```python
from build123d import *

# Parameters (mm, degrees)
F0_W     = 50.8
F0_H     = 50.8
F1_DEPTH = 6.35
F2_W     = 6.3624648929
F2_H     = 50.8
F2_W_2   = 6.35
F3_DEPTH = 44.45
F4_R     = 5.08
F5_DEPTH = 6.35
F7_DEPTH = 148.336
F8_R     = 7.9375
F9_DEPTH = 94.742


with BuildPart() as f1:
    # F0 (on Front) → F1 (new body)
    with BuildSketch(Plane.XZ):
        with Locations((-25.4, 25.4)):
            Rectangle(F0_W, F0_H)
    extrude(amount=F1_DEPTH)

    # F2 (on face) → F3 (join)
    with BuildSketch(Plane.XZ.offset(6.35)):
        with Locations((-47.6187675536, 25.4)):
            Rectangle(F2_W, F2_H)
        with Locations((-3.175, 25.4)):
            Rectangle(F2_W_2, F2_H)
    extrude(amount=F3_DEPTH)

    # F4
    f4_edges = [f1.edges().sort_by_distance(p)[0] for p in [
        (-6.35, -6.35, 25.4),
        (-50.8, 0, 25.4),
        (-44.437535, -6.35, 25.4),
        (0, 0, 25.4),
    ]]
    fillet(f4_edges, radius=F4_R)

    # F5 (add): faces of the model
    f5_faces = [f1.faces().sort_by_distance(p)[0] for p in [
        (-47.6187675536, -50.8, 25.4),
        (-3.175, -50.8, 25.4),
        (-47.6187675536, -50.8, 25.4),
        (-3.175, -50.8, 25.4),
    ]]
    extrude(f5_faces, amount=F5_DEPTH)

    # F6 (on face) → F7 (cut)
    with BuildSketch(Plane(origin=(-50.8, 0, 0), x_dir=(0, -1, 0), z_dir=(-1, 0, 0))):
        with BuildLine():
            ThreePointArc((31.115, 50.8), (49.0755122421, 43.3605122421), (56.515, 25.4))
            ThreePointArc((56.515, 25.4), (49.0755122421, 7.4394877579), (31.115, 0))
            Line((31.115, 0), (57.15, 0))
            Line((57.15, 0), (57.15, 50.8))
            Line((57.15, 50.8), (31.115, 50.8))
        make_face()
    extrude(amount=-F7_DEPTH, mode=Mode.SUBTRACT)

    # F8 (on face) → F9 (cut)
    with BuildSketch(Plane(origin=(-50.8, 0, 0), x_dir=(0, -1, 0), z_dir=(-1, 0, 0))):
        with Locations((37.0687320828, 25.4)):
            Circle(F8_R)
    extrude(amount=-F9_DEPTH, mode=Mode.SUBTRACT)


solid = f1.part
```
Design review of the part built by this model. Coordinates are the model's own, in mm. A direction names the side the tool comes from. Coordinates: 2 decimals unless noted, no trailing zeros. Loops run counter-clockwise (first coordinate to the right, second up) from the corner with the lowest first, then second, coordinate; pieces in that order, holes last.
Q1. To check wall thickness, follow line 1 (X direction, y = -35, z = 12.5); line 2 (Y direction, x = -13, z = 33); line 3 (Y direction, x = -48, z = 25). State the ranges of each line that lie inside material, in increasing order.
Reported:
line 1: x = -50.8 to -44.44, -6.35 to 0
line 2: y = -6.35 to 0
line 3: y = -56.51 to -45, -29.14 to -0.54
Q2. We need section B-B on z = 5. State the section outline as (x, y) points.
Reported:
outline: (-50.8, -46.25) - (-44.44, -46.25) - (-44.44, -11.43) arc R5.08 cw to (-39.36, -6.35) - (-11.43, -6.35) arc R5.08 cw to (-6.35, -11.43) - (-6.35, -46.25) - (0, -46.25) - (0, -5.08) arc R5.08 ccw to (-5.08, 0) - (-45.72, 0) arc R5.08 ccw to (-50.8, -5.08) - close
Q3. For pin 1 (5 mm diameter, centred on x = -41.5, z = 39.5, fed in from -Y); pin 2 (14 mm diameter, centred on x = -29, z = 33, fed in from -Y), all flat-tipped, find the tip position at first contact; note any pin that passes through.
Reported:
pin 1: stops at y = -9.37
pin 2: stops at y = -6.35
Q4. We need section C-C on x = -19.5. State the section outline as (y, z) points.
Reported:
outline: (-6.35, 0) - (0, 0) - (0, 50.8) - (-6.35, 50.8) - close
Q5. The part is to be moulded in two halves that separate along X. For faces 3 (the face through (-6.35, -28.6, 25)), 4 (the face through (-26, 0, 26)), 5 (the face through (0, -25, 25)), 6 (the face through (-7.799, -7.878, 25.756)), say which applies: +X half, -X half, draft (parallel to the pull), parting line (faces both ways), or undercut.
Reported:
face 3: undercut
face 4: draft
face 5: +X half
face 6: undercut
Q6. We need section D-D on z = 46. State the section outline as (x, y) points.
Reported:
outline: (-50.8, -45.97) - (-44.44, -45.97) - (-44.44, -11.43) arc R5.08 cw to (-39.36, -6.35) - (-11.43, -6.35) arc R5.08 cw to (-6.35, -11.43) - (-6.35, -45.97) - (0, -45.97) - (0, -5.08) arc R5.08 ccw to (-5.08, 0) - (-45.72, 0) arc R5.08 ccw to (-50.8, -5.08) - close
Q7. Tool access review of faces 1 (the face through (-26, -5, 0)), 2 (the face through (-26, -6.35, 26)): name each direction out of +Z, -Z, +X, -X, +Y, -Y from which nothing blocks a thin tool from reaching the whole face with its end or side.
Reported:
face 1: -Z, +X, -X, +Y, -Y
face 2: +Z, -Z, -Y
Q8. We need section A-A on y = -14. State the section outline as (x, z) points.
Reported:
outline: (-50.8, 0) - (-44.44, 0) - (-44.44, 50.8) - (-50.8, 50.8) - close; (-6.35, 0) - (0, 0) - (0, 50.8) - (-6.35, 50.8) - close
